Could you check a few things on this model? Use its own coordinates, in mm. Face numbers are marked on the shaded views. Round coordinates to 2 decimals unless told otherwise and drop trailing zeros. Write each loop counter-clockwise with the first axis right and the second up, starting at its lowest first coordinate (ties: lowest second). Pieces come first, ordered by that corner, then holes. Notation, with made-up numbers: (83.5, 79) -> (108.5, 79) arc R22 ccw to (108.5, 87) -> close; hole circle Ø7 at (72, -11.5). An arc over 180 degrees is marked (long way). One line per question, with ' | ' between items. Start each with the question number.
1. If I drill on line 1 along X through (y, z) = (53, 8); line 2 along Y through (x, z) = (0, -9); line 3 along Z through (x, y) = (0, 47.5), over which ranges is the centre line in solid material (lowest first)? Write a range as [from, to].
2. Imagine slicing it at A-A, the plane y = 9. List the corners of the cut face in (x, z) for me, and give its area (3 significant figures).
3. Thinking about a two-plate mould opening in X: for the marked faces 1, 2, 3 and 4, which applies, released by +X, released by -X, zero draft, split by the parting line, or undercut?
4. For pin 1 Ø6 at (x, z) = (4, -8.5) entering from -Y; pin 2 Ø1.2 at (x, z) = (0.5, -4.5) entering from -Y; pin 3 Ø2 at (x, z) = (0, 7.5) entering from -Y, each with a flat end and sliding along its axis, tell me the tip position at first contact or that it passes through.
5. Imagine slicing it at B-B, the plane y = 53. List the corners of the cut face in (x, z) for me.
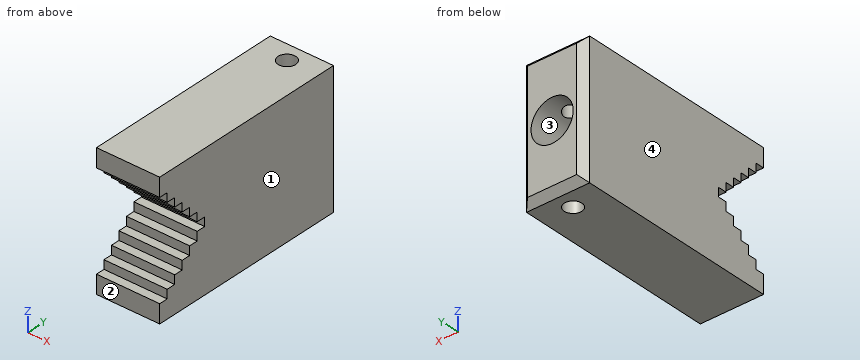
from build123d import *

# Parameters (mm, degrees)
BOSS_EXTRUDE1_DEPTH       = 9
CHAMFER1_SIZE             = 2
F_1_0MM_DOWEL_HOLE1_D     = 12
F_1_0MM_DOWEL_HOLE1_DEPTH = 18
F_1_0MM_DOWEL_HOLE1_TIP   = 3.464101615
M6X1_0_TAPPED_HOLE1_D     = 5


with BuildPart() as part:
    # Sketch1 → Boss-Extrude1 (new, symmetric)
    with BuildSketch(Plane(origin=(0, 0, 0), x_dir=(0, 0, -1), z_dir=(1, 0, 0))):
        Polygon((19, 60), (-19, 60), (-19, 0), (-13.75, 0), (-13.75, 2.5), (-11.25, 2.5), (-11.25, 5), (-8.75, 5), (-8.75, 7.5), (-6.25, 7.5), (-6.25, 10), (-3.75, 10), (-3.75, 12.5), (-1.25, 12.5), (-1.25, 15), (1.25, 15), (1.25, 12.5), (3.75, 12.5), (3.75, 10), (6.25, 10), (6.25, 7.5), (8.75, 7.5), (8.75, 5), (11.25, 5), (11.25, 2.5), (13.75, 2.5), (13.75, 0), (19, 0), align=None)
    extrude(amount=BOSS_EXTRUDE1_DEPTH, both=True)

    # Chamfer1
    chamfer1_edges = [part.edges().sort_by_distance(p)[0] for p in [
        (-9, 60, 0),
        (0, 60, 19),
        (0, 60, -19),
        (9, 60, 0),
    ]]
    chamfer(chamfer1_edges, length=CHAMFER1_SIZE)

    # Ø1.0mm Dowel Hole1
    with Locations(Plane(origin=(0, 60, 0), x_dir=(1, 0, 0), z_dir=(0, 1, 0))):
        with Locations((0, 0)):
            Hole(F_1_0MM_DOWEL_HOLE1_D / 2, depth=F_1_0MM_DOWEL_HOLE1_DEPTH)
            with Locations((0, 0, -(F_1_0MM_DOWEL_HOLE1_DEPTH + F_1_0MM_DOWEL_HOLE1_TIP / 2))):  # 120° drill point
                Cone(0, F_1_0MM_DOWEL_HOLE1_D / 2, F_1_0MM_DOWEL_HOLE1_TIP, mode=Mode.SUBTRACT)

    # M6x1.0 Tapped Hole1 (through all)
    with Locations(Plane.XY.offset(19)):
        with Locations((0, 53)):
            Hole(M6X1_0_TAPPED_HOLE1_D / 2)


solid = part.part
Geometry results:
1) line 1: x = [-9, -2.5], [2.5, 9] | line 2: y = [5, 50.5], [55.5, 60] | line 3: z = [-19, -6], [6, 19]
2) outline: (-9, -19) -> (9, -19) -> (9, -6.25) -> (-9, -6.25) -> close; (-9, 6.25) -> (9, 6.25) -> (9, 19) -> (-9, 19) -> close | area: 459 mm2
3) face 1: released by +X | face 2: zero draft | face 3: undercut | face 4: released by -X
4) pin 1: stops at y = 2.5 | pin 2: stops at y = 10 | pin 3: stops at y = 7.5
5) outline: (-9, -19) -> (-2.5, -19) -> (-2.5, -5.45) arc R6 cw to (-2.5, 5.45) -> (-2.5, 19) -> (-9, 19) -> close; (2.5, -19) -> (9, -19) -> (9, 19) -> (2.5, 19) -> (2.5, 5.45) arc R6 cw to (2.5, -5.45) -> close
